Work out the finished part from the listing and answer in its coordinate system (mm). A direction names the side the tool comes from. Give positions to 0.01 mm unless a question says otherwise; leave off trailing zeros. Loops run counter-clockwise (first coordinate to the right, second up) from the corner with the lowest first, then second, coordinate; pieces in that order, holes last. Notation, with made-up numbers: (-14, 2.25) -> (16, 2.25) arc R15 ccw to (16, 12.25) -> close; hole circle Ø4 at (17, 26). An arc over 180 degrees is marked (long way). Answer as CSV lines item,"result". Start each with the question number.
1. Find section C-C, the plane x = 11.5. Give the vertices of the cut face in (y, z), and give its area (3 significant figures).
2. Determine the mould class of faces 4 (the face through (-41.724, 0, 0)), 5 (the face through (8.737, -3.289, 10.444)), 6 (the face through (-19.734, -7.187, -5.916)) for opening direction Y: +Y half, -Y half, draft (parallel to the pull), parting line (faces both ways), or undercut.
3. Find the intervals of material crossed by line 1 along X through (y, z) = (9.75, 3); line 2 along Y through (x, z) = (20.5, 9.75); line 3 along X through (y, z) = (-3.25, -0.25), in increasing order.
4. A tool of negligible diameter and unlimited length cuts with its end or side. For faces 1 (the face through (-6.644, 10, -5)), 2 (the face through (-35, -2, 0)), 3 (the face through (-37.534, 1.397, -0.087)), from which of +Z, -Z, +X, -X, +Y, -Y can it reach the whole face along a straight path? Write none if from no direction.
5. Find section B-B, the plane z = 0. Give the vertices of the cut face in (x, y) (3 decimals).
6. Find section D-D, the plane x = -23. Give the vertices of the cut face in (y, z) (3 decimals).
7. Find section A-A, the plane y = 0. Give the vertices of the cut face in (x, z) (3 decimals).
8. Flat-ended cylindrical pins translate along their axes: pin 1 Ø1.6 at (y, z) = (-6.5, -6) entering from -X; pin 2 Ø12 at (x, y) = (-23, -3) entering from -Z (3 decimals); pin 3 Ø3 at (x, y) = (-5.5, 1.5) entering from +Z; pin 4 Ø10 at (x, y) = (15.5, -7.5) entering from +Z. Find the tip coordinate at first contact, or state that the pin passes through.
from build123d import *

# Parameters (mm, degrees)
CUT_EXTRUDE1_DEPTH = 8.5
SKETCH4_R          = 1
CUT_EXTRUDE2_DEPTH = 10


with BuildPart() as part:
    # Sketch2 → Revolve1 (revolve)
    with BuildSketch(Plane(origin=(0, 0, 0), x_dir=(1, 0, 0), z_dir=(0, 1, 0)), mode=Mode.PRIVATE) as revolve1_sk:
        Polygon((-41.724352159, 0), (24.555647841, 0), (24.555647841, 10.95), (-6.644352159, 10.95), (-6.644352159, 11.965), (-24.664352159, 11.965), (-24.664352159, 4.97), (-27.494352159, 4.97), (-27.494352159, 3.965), (-28.224352159, 3.965), (-28.224352159, 3.2), (-28.824352159, 3.2), (-28.824352159, 2), (-41.724352159, 2), align=None)
    revolve(revolve1_sk.sketch.rotate(Axis((-41.724352159, 0, 0), (1, 0, 0)), 180), axis=Axis((-41.724352159, 0, 0), (1, 0, 0)))

    # Sketch3 → Cut-Extrude1 (cut)
    with BuildSketch(Plane.ZY.offset(41.724352159)):
        with BuildLine():
            Line((-1.493929209, 1.329727611), (1.359340223, 1.467035841))
            ThreePointArc((1.359340223, 1.467035841), (-0.096134989, 1.99768818), (-1.493929209, 1.329727611))
        make_face()
    extrude(amount=-CUT_EXTRUDE1_DEPTH, mode=Mode.SUBTRACT)

    # Sketch4 → Cut-Extrude2 (cut)
    with BuildSketch(Plane.ZY.offset(24.664352159)):
        with Locations((-2.529015446, 8.04098341)):
            Circle(SKETCH4_R)
        with Locations((-5.699188182, -6.210683328)):
            Circle(SKETCH4_R)
        with Locations((8.228203628, -1.830300082)):
            Circle(SKETCH4_R)
    extrude(amount=-CUT_EXTRUDE2_DEPTH, mode=Mode.SUBTRACT)


solid = part.part
Resolved:
1,outline,"circle Ø21.9 at (0, 0)"
1,area,"377 mm^2"
2,face 4,"draft"
2,face 5,"parting line"
2,face 6,"undercut"
3,line 1,"x = -24.66 to 24.56"
3,line 2,"y = -4.98 to 4.98"
3,line 3,"x = -28.22 to 24.56"
4,face 1,"+X"
4,face 2,"-X"
4,face 3,"-Z, -X, +Y"
5,outline,"(-41.724, -2) -> (-28.824, -2) -> (-28.824, -3.2) -> (-28.224, -3.2) -> (-28.224, -3.965) -> (-27.494, -3.965) -> (-27.494, -4.97) -> (-24.664, -4.97) -> (-24.664, -11.965) -> (-6.644, -11.965) -> (-6.644, -10.95) -> (24.556, -10.95) -> (24.556, 10.95) -> (-6.644, 10.95) -> (-6.644, 11.965) -> (-24.664, 11.965) -> (-24.664, 4.97) -> (-27.494, 4.97) -> (-27.494, 3.965) -> (-28.224, 3.965) -> (-28.224, 3.2) -> (-28.824, 3.2) -> (-28.824, 2) -> (-33.224, 2) -> (-33.224, 1.402) -> (-41.724, 1.402) -> close"
6,outline,"circle Ø23.93 at (0, 0); hole circle Ø2 at (-6.211, -5.699); hole circle Ø2 at (-1.83, 8.228); hole circle Ø2 at (8.041, -2.529)"
7,outline,"(-41.724, -2) -> (-28.824, -2) -> (-28.824, -3.2) -> (-28.224, -3.2) -> (-28.224, -3.965) -> (-27.494, -3.965) -> (-27.494, -4.97) -> (-24.664, -4.97) -> (-24.664, -11.965) -> (-6.644, -11.965) -> (-6.644, -10.95) -> (24.556, -10.95) -> (24.556, 10.95) -> (-6.644, 10.95) -> (-6.644, 11.965) -> (-24.664, 11.965) -> (-24.664, 4.97) -> (-27.494, 4.97) -> (-27.494, 3.965) -> (-28.224, 3.965) -> (-28.224, 3.2) -> (-28.824, 3.2) -> (-28.824, 2) -> (-41.724, 2) -> close"
8,pin 1,"stops at x = -24.66"
8,pin 2,"stops at z = -11.965"
8,pin 3,"stops at z = 11.95"
8,pin 4,"stops at z = 10.66"
